```python
from build123d import *

# Parameters (mm, degrees)
BOSS_EXTRUDE1_DEPTH = 0.01
BOSS_EXTRUDE2_DEPTH = 0.64
CUT_EXTRUDE1_START  = 0.64
CUT_EXTRUDE1_DEPTH  = 0.32
SKETCH4_W           = 0.65
SKETCH4_H           = 2.6
BOSS_EXTRUDE3_DEPTH = 0.32


with BuildPart() as part:
    # Sketch1 → Revolve1 (revolve)
    with BuildSketch(Plane.XY):
        with BuildLine():
            Line((0, 6.3), (-2.75, 6.3))
            ThreePointArc((-2.75, 6.3), (-3.032842712, 6.182842712), (-3.15, 5.9))
            Line((-3.15, 5.9), (-3.15, 1))
            ThreePointArc((-3.15, 1), (-3.091421356, 0.858578644), (-2.95, 0.8))
            Line((-2.95, 0.8), (-2.95, 0.6))
            ThreePointArc((-2.95, 0.6), (-3.091421356, 0.541421356), (-3.15, 0.4))
            Line((-3.15, 0.4), (-3.15, 0))
            Line((-3.15, 0), (0, 0))
            Line((0, 0), (0, 6.3))
        make_face()
    revolve(axis=Axis((0, 8.082229881, 0), (0, -1, 0)))

    # Sketch2 → Boss-Extrude1 (add)
    with BuildSketch(Plane(origin=(0, 6.3, 0), x_dir=(1, 0, 0), z_dir=(0, 1, 0))):
        with BuildLine():
            Line((-2.436570336, 1.275), (2.436570336, 1.275))
            ThreePointArc((2.436570336, 1.275), (0, 2.75), (-2.436570336, 1.275))
        make_face()
    extrude(amount=BOSS_EXTRUDE1_DEPTH)

    # Sketch3 → Boss-Extrude2 (add)
    with BuildSketch(Plane(origin=(0, 0, 0), x_dir=(-1, 0, 0), z_dir=(0, -1, 0))):
        Polygon((1.885786438, -3.3), (3.3, -1.885786438), (3.3, 3.3), (-3.3, 3.3), (-3.3, -1.885786438), (-1.885786438, -3.3), align=None)
    extrude(amount=BOSS_EXTRUDE2_DEPTH)

    # Sketch3<3> → Cut-Extrude1 (cut)
    with BuildSketch(Plane(origin=(0, 0, 0), x_dir=(-1, 0, 0), z_dir=(0, -1, 0)).offset(CUT_EXTRUDE1_START)):
        with BuildLine():
            Line((0.325, 0.9), (0.325, 3.13318927))
            ThreePointArc((0.325, 3.13318927), (0, 3.15), (-0.325, 3.13318927))
            Line((-0.325, 3.13318927), (-0.325, 0.9))
            Line((-0.325, 0.9), (0.325, 0.9))
        make_face()
        with BuildLine():
            ThreePointArc((-0.325, -3.13318927), (0, -3.15), (0.325, -3.13318927))
            Line((0.325, -3.13318927), (0.325, -0.9))
            Line((0.325, -0.9), (-0.325, -0.9))
            Line((-0.325, -0.9), (-0.325, -3.13318927))
        make_face()
        with BuildLine():
            Line((0.325, 3.13318927), (0.325, 3.3))
            Line((0.325, 3.3), (-0.325, 3.3))
            Line((-0.325, 3.3), (-0.325, 3.13318927))
            ThreePointArc((-0.325, 3.13318927), (0, 3.15), (0.325, 3.13318927))
        make_face()
        with BuildLine():
            Line((-0.325, -3.3), (0.325, -3.3))
            Line((0.325, -3.3), (0.325, -3.13318927))
            ThreePointArc((0.325, -3.13318927), (0, -3.15), (-0.325, -3.13318927))
            Line((-0.325, -3.13318927), (-0.325, -3.3))
        make_face()
    extrude(amount=-CUT_EXTRUDE1_DEPTH, mode=Mode.SUBTRACT)

    # Sketch4 → Boss-Extrude3 (add)
    with BuildSketch(Plane.XZ.offset(0.32)):
        with Locations((0, -2.2)):
            Rectangle(SKETCH4_W, SKETCH4_H)
        with Locations((0, 2.2)):
            Rectangle(SKETCH4_W, SKETCH4_H)
    extrude(amount=BOSS_EXTRUDE3_DEPTH)


solid = part.part
```
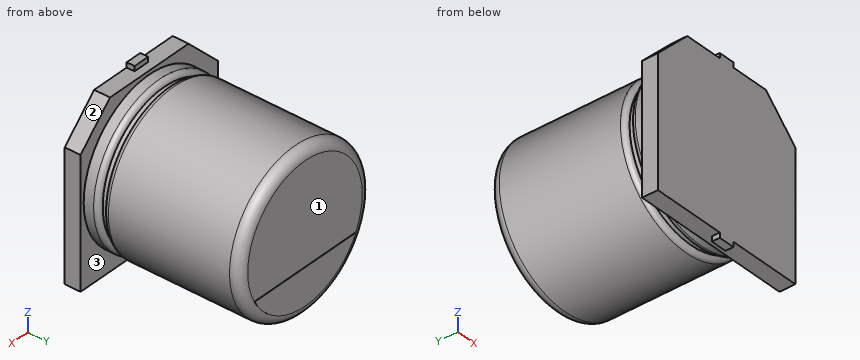
Work out the finished part from the listing and answer in its coordinate system (mm). Face numbers are marked on the shaded views. A direction names the side the tool comes from. Coordinates: 2 decimals unless noted, no trailing zeros. Write each loop counter-clockwise with the first axis right and the second up, starting at its lowest first coordinate (ties: lowest second). Pieces come first, ordered by that corner, then holes.
Q1. Which of the six approach directions +Z, -Z, +X, -X, +Y, -Y give full straight-line access (tool end or side, diameter ignored) to the marked faces 1, 2 and 3?
Q2. Find the intervals of material crossed by line 1 (Y direction, x = 1.25, z = 1.75); line 2 (Y direction, x = 2.5, z = -2.5); line 3 (X direction, y = 4, z = -1), in increasing order.
Q3. A cutting plane is placed at A-A, the plane x = 0. Give the vertices of the cut face in (y, z) (3 decimals), then the cut area to 3 significant figures.
Q4. A cutting plane is placed at C-C, the plane y = 2. Give the vertices of the cut face in (x, z).
Q5. Each of these flat-tipped pins is pushed along its axis until it touches: pin 1 Ø2 at (x, z) = (-1, 0) entering from +Y; pin 2 Ø1.5 at (x, y) = (2, 4) entering from +Z; pin 3 Ø0.5 at (x, y) = (0.5, -0.5) entering from +Z; pin 4 Ø1.5 at (x, y) = (1.5, 3.5) entering from +Z. Where does it stop, or does it pass through?
Q6. A cutting plane is placed at B-B, the plane z = 0. Give the vertices of the cut face in (x, y), then the cut area to 3 significant figures.
Findings below:
1. face 1: +Z, +X, -X, +Y
1. face 2: +Z, +X, +Y, -Y
1. face 3: +Y
2. line 1: y = -0.64 to 6.3
2. line 2: y = -0.64 to 0
2. line 3: x = -2.99 to 2.99
3. outline: (-0.64, -3.5) - (-0.32, -3.5) - (-0.32, -3.3) - (0, -3.3) - (0, -3.15) - (0.4, -3.15) arc R0.2 ccw to (0.6, -2.95) - (0.8, -2.95) arc R0.2 ccw to (1, -3.15) - (5.9, -3.15) arc R0.4 ccw to (6.3, -2.75) - (6.31, -2.75) - (6.31, -1.275) - (6.3, -1.275) - (6.3, 2.75) arc R0.4 ccw to (5.9, 3.15) - (1, 3.15) arc R0.2 ccw to (0.8, 2.95) - (0.6, 2.95) arc R0.2 ccw to (0.4, 3.15) - (0, 3.15) - (0, 3.3) - (-0.32, 3.3) - (-0.32, 3.5) - (-0.64, 3.5) - close
3. area: 43.9 mm2
4. outline: circle Ø6.3 at (0, 0)
5. pin 1: stops at y = 6.3
5. pin 2: stops at z = 2.89
5. pin 3: stops at z = 3.5
5. pin 4: stops at z = 3.06
6. outline: (-3.3, -0.64) - (3.3, -0.64) - (3.3, 0) - (3.15, 0) - (3.15, 0.4) arc R0.2 ccw to (2.95, 0.6) - (2.95, 0.8) arc R0.2 ccw to (3.15, 1) - (3.15, 5.9) arc R0.4 ccw to (2.75, 6.3) - (-2.75, 6.3) arc R0.4 ccw to (-3.15, 5.9) - (-3.15, 1) arc R0.2 ccw to (-2.95, 0.8) - (-2.95, 0.6) arc R0.2 ccw to (-3.15, 0.4) - (-3.15, 0) - (-3.3, 0) - close
6. area: 43.7 mm2
